The listing builds one solid part. Answer for the finished solid, in the listing's coordinates (mm). A direction names the side the tool comes from. Give positions to 0.01 mm unless a question says otherwise; leave off trailing zeros. Order: outer loops, then holes, each group sorted by start corner. A loop starts at its lowest first (then second) coordinate and runs counter-clockwise, first axis right, second up. Notation, with made-up numbers: (-35.75, 49.5) - (-21.75, 49.5) arc R27 ccw to (-21.75, 75.5) - close; hole circle Ø5 at (-34, 65.5). An arc over 180 degrees is marked (long way). Answer as CSV lines item,"result". Start each with the question number.
1. Section B-B on x = 23 is taken. Give the vertices of the cut face in (y, z), and give its area (3 significant figures).
2. Consider line 1 along Z through (x, y) = (37.5, 40); line 2 along Z through (x, y) = (6.5, 10); line 3 along X through (y, z) = (36, 4.25). Determine where each line is inside the solid, lowest interval first. Write a range as [from, to].
3. Section A-A on y = 29 is taken. Give the vertices of the cut face in (x, z).
4. Which of the six approach directions +Z, -Z, +X, -X, +Y, -Y give full straight-line access (tool end or side, diameter ignored) to faces 1 (the flat face through (30.996, 33, 4)), 2 (the cylindrical face through (31.57, 33.56, 0.6)), 3 (the cylindrical face through (31.57, 33.37, 8.4)), 4 (the cylindrical face through (27.2, 16.32, 8.43)), 5 (the flat face through (6.167, -2.245, 6.437))?
5. Flat-ended cylindrical pins translate along their axes: pin 1 (4 mm diameter, centred on x = 9.5, z = 6, fed in from +Y); pin 2 (4 mm diameter, centred on x = 27.5, z = 3, fed in from -Y); pin 3 (4 mm diameter, centred on x = 28, z = 6, fed in from +Y). Find the tip coordinate at first contact, or state that the pin passes through.
6. Determine the mould class of faces 6 (the cylindrical face through (11.028, 5.744, 8.43)), 7 (the cylindrical face through (30.43, 25.32, 4.54)), 8 (the cylindrical face through (35.53, 43.43, 1.35)), 9 (the cylindrical face through (6.233, 5.601, 1.986)) for opening direction X: +X half, -X half, draft (parallel to the pull), parting line (faces both ways), or undercut.
from build123d import *

# Parameters (mm, degrees)
Y_KSEKLIK_EKSTR_ZYON1_DEPTH = 9
RADYUS1_R                   = 4.5
IZIM2_R                     = 2
KES_EKSTR_ZYON1_DEPTH       = 9
IZIM3_R                     = 2.575
KES_EKSTR_ZYON2_DEPTH       = 15
RADYUS2_R                   = 2


with BuildPart() as part:
    # Çizim1 → Yükseklik-Ekstrüzyon1 (new body)
    with BuildSketch(Plane.XY):
        Polygon((0, 0), (8.99576861, 24.715671126), (30.99576861, 24.715671126), (30.99576861, 44.715671126), (39.99576861, 44.715671126), (39.99576861, 15.715671126), (15.297636454, 15.715671126), (8.457233587, -3.07818129), align=None)
    extrude(amount=Y_KSEKLIK_EKSTR_ZYON1_DEPTH)

    # Radyus1
    radyus1_edges = [part.edges().sort_by_distance(p)[0] for p in [
        (35.49576861, 44.715671126, 0),
        (35.49576861, 44.715671126, 9),
    ]]
    fillet(radyus1_edges, radius=RADYUS1_R - 0.0001)  # a hair under: the kernel refuses the full size

    # Çizim2 → Kes-Ekstrüzyon1 (cut)
    with BuildSketch(Plane(origin=(39.99576861, 0, 0), x_dir=(0, 0, -1), z_dir=(1, 0, 0))):
        with Locations(Location((-4.5, 40.215671126, 0), (0, 0, 90))):
            Circle(IZIM2_R)
    extrude(amount=-KES_EKSTR_ZYON1_DEPTH, mode=Mode.SUBTRACT)

    # Çizim3 → Kes-Ekstrüzyon2 (cut)
    with BuildSketch(Plane(origin=(0, 0, 0), x_dir=(0.9396926207859082, -0.34202014332566943, 0), z_dir=(-0.34202014332566943, -0.9396926207859082, 0))):
        with Locations((4.5, 4.5)):
            Circle(IZIM3_R)
    extrude(amount=-KES_EKSTR_ZYON2_DEPTH, mode=Mode.SUBTRACT)

    # Radyus2
    radyus2_edges = [part.edges().sort_by_distance(p)[0] for p in [
        (27.646702532, 15.715671126, 9),
        (11.87743502, 6.318744918, 0),
        (39.99576861, 27.965721126, 9),
        (8.99576861, 24.715671126, 4.5),
        (30.99576861, 24.715671126, 4.5),
        (39.99576861, 15.715671126, 4.5),
        (15.297636454, 15.715671126, 4.5),
        (19.99576861, 24.715671126, 9),
        (30.99576861, 32.465721126, 0),
        (30.99576861, 32.465721126, 9),
        (30.99576861, 43.39768093, 7.682009805),
        (30.99576861, 43.39768093, 1.317990195),
        (4.497884305, 12.357835563, 9),
        (39.99576861, 43.39768093, 7.682009805),
        (39.99576861, 43.39768093, 1.317990195),
        (11.87743502, 6.318744918, 9),
        (4.497884305, 12.357835563, 0),
        (19.99576861, 24.715671126, 0),
        (39.99576861, 27.965721126, 0),
        (27.646702532, 15.715671126, 0),
    ]]
    fillet(radyus2_edges, radius=RADYUS2_R)


solid = part.part
Checks:
1,outline,"(15.72, 2) arc R2 ccw to (17.72, 0) - (22.72, 0) arc R2 ccw to (24.72, 2) - (24.72, 7) arc R2 ccw to (22.72, 9) - (17.72, 9) arc R2 ccw to (15.72, 7) - close"
1,area,"77.6 mm²"
2,line 1,"z = [0, 2.51], [6.49, 9]"
2,line 2,"z = [0, 2.67], [6.33, 9]"
2,line 3,"x = [31, 40]"
3,outline,"(31, 2) arc R2 ccw to (33, 0) - (38, 0) arc R2 ccw to (40, 2) - (40, 7) arc R2 ccw to (38, 9) - (33, 9) arc R2 ccw to (31, 7) - close"
4,face 1,"+Z, -Z, -X, +Y"
4,face 2,"-Z, -X, +Y"
4,face 3,"+Z, -X, +Y"
4,face 4,"+Z, +X, -Y"
4,face 5,"+Z, -Z, -X, -Y"
5,pin 1,"stops at y = 24.72"
5,pin 2,"stops at y = 15.72"
5,pin 3,"stops at y = 24.99"
6,face 6,"+X half"
6,face 7,"-X half"
6,face 8,"draft"
6,face 9,"undercut"
